The model under review builds one solid part; all positions refer to its coordinate system, in mm. Face numbers are marked on the shaded views. A direction names the side the tool comes from. Coordinates: 2 decimals unless noted, no trailing zeros. Loops run counter-clockwise (first coordinate to the right, second up) from the corner with the lowest first, then second, coordinate; pieces in that order, holes last. Notation, with made-up numbers: (60, -17) - (116, -17) arc R22 cw to (116, 2) - close; hole circle Ø6 at (39.5, 88.5). An arc over 180 degrees is marked (long way). Use a Markdown table: item, result. Add a question column.
1) Add section D-D, the plane z = 37. Give the boundary of the cut face in (x, y), and give its area (3 significant figures).
2) Clearance check with flat-ended pins moving along their axes: pin 1 (6.5 mm diameter, centred on x = -8.27, y = 24.77, fed in from -Z); pin 2 (1.5 mm diameter, centred on x = -15.5, y = 27.5, fed in from -Z); pin 3 (6 mm diameter, centred on x = -33, z = 10, fed in from +Y); pin 4 (3 mm diameter, centred on x = -13.5, z = 26.5, fed in from -Y). State where each tip first meets the part, or that it passes through.
3) The part is to be moulded in two halves that separate along X. For the marked faces 1, 2 and 3, say which applies: pulls with the +X half, pulls with the -X half, needs draft (parallel to the pull), parting line crosses it, or undercut.
4) Add section B-B, the plane y = 37.5. Give the boundary of the cut face in (x, z).
5) For the marked faces 4 and 5, list the 3-axis set-ups (+Z, -Z, +X, -X, +Y, -Y) from which the entire face can be reached by the end or side of a thin tool; tool diameter is ignored.
6) Add section A-A, the plane x = -21. Give the boundary of the cut face in (y, z).
7) To check wall thickness, follow L1, parallel to X at y = 2.5, z = 10; L2, parallel to X at y = 9.5, z = 39.5; L3, parallel to Y at x = -21, z = 43.2. State the ranges of each line that lie inside material, in increasing order. Write a range as [from, to].
8) Add section C-C, the plane z = 10. Give the boundary of the cut face in (x, y), and give its area (3 significant figures).
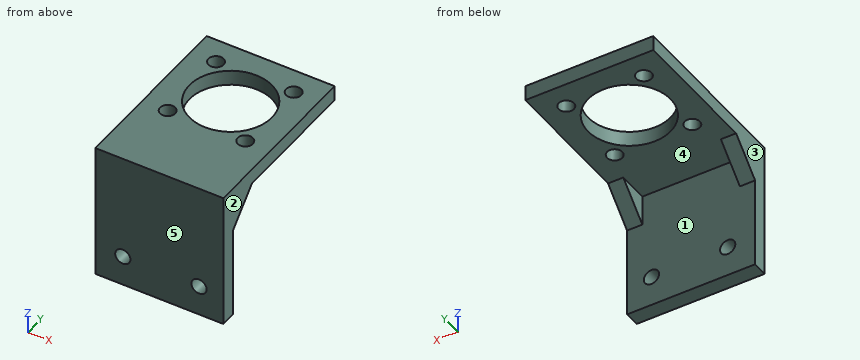
```python
from build123d import *

# Parameters (mm, degrees)
SKETCH_1_W             = 40
SKETCH_1_H             = 42
SKETCH_1_R             = 2.5
EXTRUDE_1_DEPTH        = 5
SKETCH_2_W             = 42
SKETCH_2_H             = 58.5
SKETCH_2_R             = 13.55
SKETCH_2_R_2           = 2.5
EXTRUDE_2_DEPTH        = 5
EXTRUDE_3_DEPTH        = 5
PATTERN_LINEAR_1_COUNT = 2
PATTERN_LINEAR_1_PITCH = 37


with BuildPart() as part:
    # 草图1 → 凸台-拉伸1 (new body)
    with BuildSketch(Plane(origin=(0, 0, 0), x_dir=(0, 0, -1), z_dir=(0, 1, 0))):
        with Locations((-20, 21)):
            Rectangle(SKETCH_1_W, SKETCH_1_H)
        with Locations(Location((-10, 33, 0), (0, 0, 180))):
            Circle(SKETCH_1_R, mode=Mode.SUBTRACT)
        with Locations(Location((-10, 8, 0), (0, 0, 180))):
            Circle(SKETCH_1_R, mode=Mode.SUBTRACT)
    extrude(amount=EXTRUDE_1_DEPTH)

    # 草图2 → 凸台-拉伸2 (add)
    with BuildSketch(Plane.XY.offset(40)):
        with Locations((-21, 29.25)):
            Rectangle(SKETCH_2_W, SKETCH_2_H)
        with Locations((-21, 37.5)):
            Circle(SKETCH_2_R, mode=Mode.SUBTRACT)
        with Locations((-33.727922061, 24.772077939)):
            Circle(SKETCH_2_R_2, mode=Mode.SUBTRACT)
        with Locations((-8.272077939, 50.227922061)):
            Circle(SKETCH_2_R_2, mode=Mode.SUBTRACT)
        with Locations((-33.727922061, 50.227922061)):
            Circle(SKETCH_2_R_2, mode=Mode.SUBTRACT)
        with Locations((-8.272077939, 24.772077939)):
            Circle(SKETCH_2_R_2, mode=Mode.SUBTRACT)
    extrude(amount=EXTRUDE_2_DEPTH)

    # 草图3 → 凸台-拉伸3 (add)
    with BuildSketch(Plane(origin=(0, 0, 0), x_dir=(0, 0, -1), z_dir=(1, 0, 0))):
        Polygon((-40, 15), (-40, 5), (-30, 5), align=None)
    extrude_3 = extrude(amount=-EXTRUDE_3_DEPTH)

    # 阵列(线性)1: 凸台-拉伸3 ×2
    with Locations(*[(-i * PATTERN_LINEAR_1_PITCH, 0, 0) for i in range(1, PATTERN_LINEAR_1_COUNT)]):
        add(extrude_3)


solid = part.part
```
From the geometry:
| question | item | result |
|---|---|---|
| 1 | outline | (-42, 0) - (0, 0) - (0, 12) - (-5, 12) - (-5, 5) - (-37, 5) - (-37, 12) - (-42, 12) - close |
| 1 | area | 280 mm^2 |
| 2 | pin 1 | stops at z = 40 |
| 2 | pin 2 | passes through |
| 2 | pin 3 | stops at y = 5 |
| 2 | pin 4 | stops at y = 0 |
| 3 | face 1 | undercut |
| 3 | face 2 | pulls with the +X half |
| 3 | face 3 | pulls with the -X half |
| 4 | outline | (-42, 40) - (-34.55, 40) - (-34.55, 45) - (-42, 45) - close; (-7.45, 40) - (0, 40) - (0, 45) - (-7.45, 45) - close |
| 5 | face 4 | -Z, +Y |
| 5 | face 5 | +Z, -Z, +X, -X, -Y |
| 6 | outline | (0, 0) - (5, 0) - (5, 40) - (23.95, 40) - (23.95, 45) - (0, 45) - close; (51.05, 40) - (58.5, 40) - (58.5, 45) - (51.05, 45) - close |
| 7 | L1 | x = [-42, -35.5], [-30.5, -10.5], [-5.5, 0] |
| 7 | L2 | x = [-42, -37], [-5, 0] |
| 7 | L3 | y = [0, 23.95], [51.05, 58.5] |
| 8 | outline | (-42, 0) - (-35.5, 0) - (-35.5, 5) - (-42, 5) - close; (-30.5, 0) - (-10.5, 0) - (-10.5, 5) - (-30.5, 5) - close; (-5.5, 0) - (0, 0) - (0, 5) - (-5.5, 5) - close |
| 8 | area | 160 mm^2 |
